Here's how the part is built. I have some questions about the finished solid (model axes, mm). Give positions to 0.01 mm unless a question says otherwise; leave off trailing zeros. Order: outer loops, then holes, each group sorted by start corner. A loop starts at its lowest first (then second) coordinate and runs counter-clockwise, first axis right, second up.
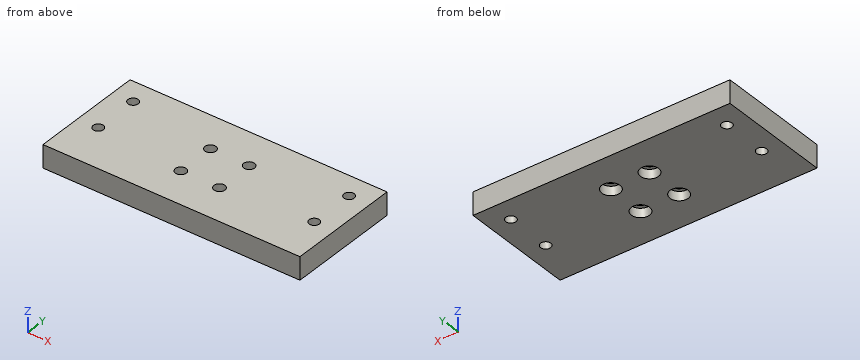
from build123d import *

# Parameters (mm, degrees)
SKETCH1_W                      = 113
SKETCH1_H                      = 50
BOSS_EXTRUDE1_DEPTH            = 10
CBORE_FOR_M4_SHCS1_D           = 4.8
CBORE_FOR_M4_SHCS1_CBORE_D     = 8
CBORE_FOR_M4_SHCS1_CBORE_DEPTH = 4
SKETCH4_R                      = 2.25
CUT_EXTRUDE1_DEPTH             = 63.587938135


with BuildPart() as part:
    # Sketch1 → Boss-Extrude1 (new body)
    with BuildSketch(Plane.XY):
        Rectangle(SKETCH1_W, SKETCH1_H)
    extrude(amount=BOSS_EXTRUDE1_DEPTH)

    # CBORE for M4 SHCS1 (through all)
    with Locations(Plane(origin=(0, 0, 0), x_dir=(-1, 0, 0), z_dir=(0, 0, -1))):
        with Locations((-8.5, 8.5), (-8.5, -8.5), (8.5, -8.5), (8.5, 8.5)):
            CounterBoreHole(CBORE_FOR_M4_SHCS1_D / 2, CBORE_FOR_M4_SHCS1_CBORE_D / 2, CBORE_FOR_M4_SHCS1_CBORE_DEPTH)

    # Sketch4 → Cut-Extrude1 (cut, through all)
    with BuildSketch(Plane(origin=(0, 0, 0), x_dir=(-1, 0, 0), z_dir=(0, 0, -1))):
        with Locations((-47.5, 15)):
            Circle(SKETCH4_R)
        with Locations((-47.5, -5)):
            Circle(SKETCH4_R)
        with Locations(Location((47.5, -5, 0), (0, 0, 180))):
            Circle(SKETCH4_R)
        with Locations(Location((47.5, 15, 0), (0, 0, 180))):
            Circle(SKETCH4_R)
    extrude(amount=-CUT_EXTRUDE1_DEPTH, mode=Mode.SUBTRACT)


solid = part.part
Q1. If we section it at B-B on y = -8.5: List the corners of the cut face in (x, z) for me.
Filled sheet:
outline: (-56.5, 0) - (-12.5, 0) - (-12.5, 4) - (-10.9, 4) - (-10.9, 10) - (-56.5, 10) - close; (-6.1, 4) - (-4.5, 4) - (-4.5, 0) - (4.5, 0) - (4.5, 4) - (6.1, 4) - (6.1, 10) - (-6.1, 10) - close; (10.9, 4) - (12.5, 4) - (12.5, 0) - (56.5, 0) - (56.5, 10) - (10.9, 10) - close
Q2. I need wall thicknesses on L1, parallel to Y at x = -8.5, z = 6; L2, parallel to Y at x = 47.5, z = 6; L3, parallel to X at y = 15.5, z = 5.75. Which ranges of each line are inside material? Lowest first, please.
Filled sheet:
L1: y = -25 to -10.9, -6.1 to 6.1, 10.9 to 25
L2: y = -25 to -7.25, -2.75 to 12.75, 17.25 to 25
L3: x = -56.5 to -49.69, -45.31 to 45.31, 49.69 to 56.5
Q3. If we section it at A-A on x = -8.5: List the corners of the cut face in (y, z) for me.
Filled sheet:
outline: (-25, 0) - (-12.5, 0) - (-12.5, 4) - (-10.9, 4) - (-10.9, 10) - (-25, 10) - close; (-6.1, 4) - (-4.5, 4) - (-4.5, 0) - (4.5, 0) - (4.5, 4) - (6.1, 4) - (6.1, 10) - (-6.1, 10) - close; (10.9, 4) - (12.5, 4) - (12.5, 0) - (25, 0) - (25, 10) - (10.9, 10) - close
Q4. I'm going to push a flat-ended pin straight in: P1, Ø5, axis at x = 8.5, y = -8.5, coming from the -Z side. Where does the tip first touch, or does it pass through?
Filled sheet:
P1: stops at z = 4
Q5. If we section it at C-C on z = 2: Give the number of separate pieces and of enclosed holes in the cut face, plus the area to 3 significant figures.
Filled sheet:
separate pieces: 1
enclosed holes: 8
area: 5,390 mm2
